The model under review builds one solid part; all positions refer to its coordinate system, in mm. A direction names the side the tool comes from. Round coordinates to 2 decimals unless told otherwise and drop trailing zeros. Order: outer loops, then holes, each group sorted by start corner. A loop starts at its lowest first (then second) coordinate and runs counter-clockwise, first axis right, second up. Notation, with made-up numbers: M 57.5,22.25 L 101.5,22.25 A10 cw 101.5,41.25 Z; hole C -27.75,16 d5. An arc over 180 degrees is marked long. Answer as a JSON object with one key per item and string values. Group by question number.
1) Consider section C-C, the plane x = -17.5. Write out the cut boundary in (y, z), then the cut area to 3 significant figures.
2) Insertion check: pin 1 Ø1.3 at (x, z) = (0.5, 10) entering from -Y; pin 2 Ø1.6 at (x, z) = (2, 12) entering from +Y; pin 3 Ø4 at (x, z) = (-13, 8) entering from -Y. Each pin has a flat end and moves straight along its axis. Give the tip position at first contact, or say it passes through.
3) For faces 1 (the flat face through (-10, 3.6, 12)), 2 (the flat face through (18, -2, 2)), 3 (the flat face through (-10, -3.6, 12)), list the 3-axis set-ups (+Z, -Z, +X, -X, +Y, -Y) from which the entire face can be reached by the end or side of a thin tool; tool diameter is ignored.
4) To check wall thickness, follow line 1 (X direction, y = 0, z = 0.6); line 2 (Y direction, x = 18.5, z = 1.2). State the ranges of each line that lie inside material, in increasing order.
5) Consider section B-B, the plane x = -10. Write out the cut boundary in (y, z), then the cut area to 3 significant figures.
6) The part is to be moulded in two halves that separate along X. For faces 4 (the flat face through (6, 3.75, 12)), 5 (the flat face through (14.75, 0, 8)), 6 (the cylindrical face through (17.32, 1.08, 0.99)), say which applies: +X half, -X half, draft (parallel to the pull), parting line (faces both ways), or undercut.
7) Consider section D-D, the plane y = 0.75. Write out the cut boundary in (x, z).
8) Consider section A-A, the plane z = 12.75. Write out the cut boundary in (x, y).
```python
from build123d import *

# Parameters (mm, degrees)
SKETCH1_W               = 29.5
SKETCH1_H               = 8.4
BOSS_EXTRUDE1_DEPTH     = 11.5
SKETCH2_W               = 7.5
SKETCH2_H               = 7.2
SKETCH2_W_2             = 16.3
SKETCH2_H_2             = 7.5
BOSS_EXTRUDE2_DEPTH     = 2
SKETCH3_W               = 29.5
SKETCH3_H               = 13
BOSS_EXTRUDE3_DEPTH     = 7.2
BOSS_EXTRUDE4_DEPTH     = 5.05
SKETCH5_R               = 1.6
BOSS_EXTRUDE5_DEPTH     = 10
CUT_EXTRUDE1_START      = -8
SKETCH8_R               = 3.75
CUT_EXTRUDE1_DEPTH      = 8
CUT_EXTRUDE2_DEPTH      = 29.452811812
CUT_EXTRUDE2_DEPTH_BACK = 29.452811812


with BuildPart() as part:
    # Sketch1 → Boss-Extrude1 (new body)
    with BuildSketch(Plane.XY):
        Rectangle(SKETCH1_W, SKETCH1_H)
    extrude(amount=BOSS_EXTRUDE1_DEPTH)

    # Sketch2 → Boss-Extrude2 (add)
    with BuildSketch(Plane.XY.offset(11.5)):
        with Locations((-10.25, 0)):
            Rectangle(SKETCH2_W, SKETCH2_H)
        with Locations((5.8, 0)):
            Rectangle(SKETCH2_W_2, SKETCH2_H_2)
    extrude(amount=BOSS_EXTRUDE2_DEPTH)

    # Sketch3 → Boss-Extrude3 (add)
    with BuildSketch(Plane.XY):
        Rectangle(SKETCH3_W, SKETCH3_H)
    extrude(amount=BOSS_EXTRUDE3_DEPTH)

    # Sketch4 → Boss-Extrude4 (add, symmetric)
    with BuildSketch(Plane(origin=(0, 0, 0), x_dir=(0, 0, -1), z_dir=(1, 0, 0))):
        Polygon((-5.55, -6.5), (-5.55, -11.5), (-8.85, -11.5), (-8.85, -6.5), (-8.35, -6.5), (-7.2, -5.35), (-7.2, -6.5), align=None)
    extrude(amount=BOSS_EXTRUDE4_DEPTH, both=True)

    # Sketch5 → Boss-Extrude5 (add)
    # profile 1 of 2: a face of its own
    with BuildSketch(Plane.XY):
        with BuildLine():
            Line((-18.5, 3.75), (-14.75, 3.75))
            Line((-14.75, 3.75), (-14.75, -3.75))
            Line((-14.75, -3.75), (-18.5, -3.75))
            ThreePointArc((-18.5, -3.75), (-22.25, 0), (-18.5, 3.75))
        make_face()
        with Locations((-18.5, 0)):
            Circle(SKETCH5_R, mode=Mode.SUBTRACT)
    # profile 2 of 2: a face of its own
    with BuildSketch(Plane.XY):
        with BuildLine():
            Line((18.5, 3.75), (14.75, 3.75))
            Line((14.75, 3.75), (14.75, -3.75))
            Line((14.75, -3.75), (18.5, -3.75))
            ThreePointArc((18.5, -3.75), (22.25, 0), (18.5, 3.75))
        make_face()
        with Locations((18.5, 0)):
            Circle(SKETCH5_R, mode=Mode.SUBTRACT)
    extrude(amount=BOSS_EXTRUDE5_DEPTH)

    # Sketch8 → Cut-Extrude1 (cut)
    with BuildSketch(Plane.XY.offset(10).offset(CUT_EXTRUDE1_START)):
        with Locations((-18.5, 0)):
            Circle(SKETCH8_R)
        with Locations((18.5, 0)):
            Circle(SKETCH8_R)
    extrude(amount=CUT_EXTRUDE1_DEPTH, mode=Mode.SUBTRACT)

    # Sketch9 → Cut-Extrude2 (cut, two sides: drawn at the far end of the back side and taken through both)
    with BuildSketch(Plane(origin=(0, 0, 0), x_dir=(1, 0, 0), z_dir=(0, 1, 0)).offset(-CUT_EXTRUDE2_DEPTH_BACK)):
        Polygon((-18.5, -4), (-14.75, -7.75), (-14.75, -10), (-18.5, -10), align=None)
        Polygon((18.5, -10), (18.5, -4), (14.75, -7.75), (14.75, -10), align=None)
    extrude(amount=CUT_EXTRUDE2_DEPTH + CUT_EXTRUDE2_DEPTH_BACK, mode=Mode.SUBTRACT)


solid = part.part
```
Results list:
{
 "1": {"outline": "M -3.75,0 L -1.25,0 L -1.25,2 L -3.61,2 L -3.61,5 L -3.75,5 Z; M 1.25,0 L 3.75,0 L 3.75,5 L 3.61,5 L 3.61,2 L 1.25,2 Z", "area": "10.8 mm^2"},
 "2": {"pin 1": "y = -4.2", "pin 2": "y = 4.2", "pin 3": "y = -6.5"},
 "3": {"face 1": "+Z, -X, +Y", "face 2": "+Z, +X", "face 3": "+Z, -X, -Y"},
 "4": {"line 1": "-22.25 to -20.1, -16.9 to 16.9, 20.1 to 22.25", "line 2": "-3.75 to -1.6, 1.6 to 3.75"},
 "5": {"outline": "M -6.5,0 L 6.5,0 L 6.5,7.2 L 4.2,7.2 L 4.2,11.5 L 3.6,11.5 L 3.6,13.5 L -3.6,13.5 L -3.6,11.5 L -4.2,11.5 L -4.2,7.2 L -6.5,7.2 Z", "area": "144 mm^2"},
 "6": {"face 4": "draft", "face 5": "+X half", "face 6": "undercut"},
 "7": {"outline": "M -22.17,0 L -19.91,0 L -19.91,2 L -22.17,2 Z; M -17.09,0 L 17.09,0 L 17.09,2 L 14.83,2 L 14.83,7.67 L 14.75,7.75 L 14.75,11.5 L 13.95,11.5 L 13.95,13.5 L -2.35,13.5 L -2.35,11.5 L -6.5,11.5 L -6.5,13.5 L -14,13.5 L -14,11.5 L -14.75,11.5 L -14.75,7.75 L -14.83,7.67 L -14.83,2 L -17.09,2 Z; M 19.91,0 L 22.17,0 L 22.17,2 L 19.91,2 Z"},
 "8": {"outline": "M -14,-3.6 L -6.5,-3.6 L -6.5,3.6 L -14,3.6 Z; M -2.35,-3.75 L 13.95,-3.75 L 13.95,3.75 L -2.35,3.75 Z"}
}
